Build history of the part. All positions in model axes, mm. Face numbers are marked on the shaded views. A direction names the side the tool comes from. Round coordinates to 2 decimals unless told otherwise and drop trailing zeros. Loops run counter-clockwise (first coordinate to the right, second up) from the corner with the lowest first, then second, coordinate; pieces in that order, holes last. Notation, with made-up numbers: (76.25, 35.5) -> (80.25, 35.5) arc R15 cw to (80.25, 45.5) -> close; hole circle Ø6 at (83.5, 82.25). An arc over 180 degrees is marked (long way). Put each result on its own line as item: value. Start each with the question number.
```python
from build123d import *

# Parameters (mm, degrees)
SKETCH1_W           = 80
SKETCH1_H           = 65.45
BOSS_EXTRUDE1_DEPTH = 31
BOSS_EXTRUDE3_DEPTH = 5
CHAMFER2_SIZE       = 25
CHAMFER2_SIZE2      = 20.977490779
SHELL2_START        = -36
SHELL2_DEPTH        = 72
SHELL2_START_2      = -41
SHELL2_2_OUTLINE_W  = 1
SHELL2_2_OUTLINE_H  = 57.45
SHELL2_2_DEPTH      = 82
SKETCH6_R           = 4.86874318
CUT_EXTRUDE1_DEPTH  = 5
BOSS_EXTRUDE4_DEPTH = 8
BOSS_EXTRUDE5_REACH = 107.939
BOSS_EXTRUDE5_START = 29.5
SKETCH10_W          = 12.25
SKETCH10_H          = 9
CUT_EXTRUDE2_DEPTH  = 6
CHAMFER3_SIZE       = 2
CHAMFER3_SIZE2      = 1.865030172
CHAMFER4_SIZE       = 7.098078142
CHAMFER4_SIZE_2     = 10
CHAMFER5_SIZE       = 10
CHAMFER7_SIZE       = 5
SKETCH11_R          = 0.93
CUT_EXTRUDE3_DEPTH  = 7


# Read off the part's stored shape, not the designer's step: Shell2
with BuildPart() as part:
    # Sketch1 → Boss-Extrude1 (new body)
    with BuildSketch(Plane(origin=(0, 0, 0), x_dir=(1, 0, 0), z_dir=(0, 1, 0))):
        Rectangle(SKETCH1_W, SKETCH1_H)
    extrude(amount=BOSS_EXTRUDE1_DEPTH)

    # Sketch5 → Boss-Extrude3 (add)
    with BuildSketch(Plane.ZY.offset(40)):
        Polygon((-32.725, 31), (-20.625, 31), (8.005, 31), (32.725, 31), (32.725, 26), (2.6203214, 26), (6.0203214, 22.6), (-5.2796786, 22.6), (-1.8796786, 26), (-16.125, 26), (-12.725, 22.6), (-24.025, 22.6), (-20.625, 26), (-32.725, 26), align=None)
    boss_extrude3 = extrude(amount=BOSS_EXTRUDE3_DEPTH)

    # Mirror1: Boss-Extrude3 across plane
    add(boss_extrude3.mirror(Plane(origin=(0, 0, 0), x_dir=(0, 0, 1), z_dir=(1, 0, 0))))

    # Chamfer2
    chamfer2_edges = [part.edges().sort_by_distance(p)[0] for p in [
        (0, 0, 32.725),
    ]]
    chamfer2_side = [part.faces().sort_by_distance(p)[0] for p in [
        (0, 0, 0),
    ]]
    chamfer(chamfer2_edges, length=CHAMFER2_SIZE, length2=CHAMFER2_SIZE2, reference=chamfer2_side[0])

    # Shell2 outline → Shell2 (cut)
    with BuildSketch(Plane.YZ.offset(SHELL2_START)):
        Polygon((22.842721412, 28.725), (4, 6.269119063), (4, -28.725), (31, -28.725), (31, 28.725), align=None)
    extrude(amount=SHELL2_DEPTH, mode=Mode.SUBTRACT)

    # Shell2 2 outline → Shell2 2 (cut)
    with BuildSketch(Plane.YZ.offset(SHELL2_START_2)):
        with Locations((30.5, 0)):
            Rectangle(SHELL2_2_OUTLINE_W, SHELL2_2_OUTLINE_H)
    extrude(amount=SHELL2_2_DEPTH, mode=Mode.SUBTRACT)

    # Sketch6 → Cut-Extrude1 (cut)
    with BuildSketch(Plane(origin=(0, 4, 24.632603001), x_dir=(1, 0, 0), z_dir=(0, 1, 0))):
        with Locations(Location((22, 23.453346141, 0), (0, 0, 270))):
            Circle(SKETCH6_R)
        with Locations(Location((-22, 23.453346141, 0), (0, 0, 270))):
            Circle(SKETCH6_R)
    extrude(amount=-CUT_EXTRUDE1_DEPTH, mode=Mode.SUBTRACT)

    # Sketch7 → Boss-Extrude4 (add)
    with BuildSketch(Plane.XY.offset(-28.725)):
        Polygon((-14.5, 13.5), (14.5, 13.5), (14.5, 31), (13.5, 31), (13.5, 14.706896552), (-13.5, 14.706896552), (-13.5, 31), (-14.5, 31), align=None)
    extrude(amount=BOSS_EXTRUDE4_DEPTH)

    # Sketch8 → Boss-Extrude5 (add, up to next)
    with BuildSketch(Plane.XY.offset(-20.725).offset(BOSS_EXTRUDE5_START), mode=Mode.PRIVATE) as boss_extrude5_sk1:
        Polygon((-13.5, 14.706896552), (-13.5, 31), (-14.5, 31), (-14.5, 14.706896552), (-14.5, 13.5), (-13.5, 13.5), (13.5, 13.5), (14.5, 13.5), (14.5, 14.706896552), (14.5, 31), (13.5, 31), (13.5, 14.706896552), align=None)
    boss_extrude5_tool1 = extrude(boss_extrude5_sk1.sketch, amount=BOSS_EXTRUDE5_REACH, mode=Mode.PRIVATE) - part.part
    add(boss_extrude5_tool1.solids().sort_by_distance((14, 30.661289, 8.775))[0])

    # Sketch10 → Cut-Extrude2 (cut)
    with BuildSketch(Plane.XZ):
        with Locations((-26.125, -23.025)):
            Rectangle(SKETCH10_W, SKETCH10_H)
        with Locations((26.125, -23.025)):
            Rectangle(SKETCH10_W, SKETCH10_H)
    extrude(amount=-CUT_EXTRUDE2_DEPTH, mode=Mode.SUBTRACT)

    # Chamfer3
    chamfer3_edges = [part.edges().sort_by_distance(p)[0] for p in [
        (0, 31, -32.725),
    ]]
    chamfer3_side = [part.faces().sort_by_distance(p)[0] for p in [
        (0, 15.756916996, -32.725),
    ]]
    chamfer(chamfer3_edges, length=CHAMFER3_SIZE, length2=CHAMFER3_SIZE2, reference=chamfer3_side[0])

    # Chamfer4
    # the kernel refuses this chamfer: 10, 7.098078142 mm, written as the material it adds along each edge
    with BuildSketch(Plane(origin=(14.5, 13.5, 17.590778193), x_dir=(0, -0.6849156240265527, -0.728622390518105), z_dir=(-1, 0, 0))) as chamfer4_piece_1_section:
        Polygon((CHAMFER4_SIZE * 0.998412410217, -CHAMFER4_SIZE * 0.0563263630269), (CHAMFER4_SIZE_2 * 0.728622390518, -CHAMFER4_SIZE_2 * 0.684915624027), (0, 0), align=None)
    chamfer4_piece_1 = extrude(amount=29, mode=Mode.PRIVATE)
    chamfer4_piece_1 = split(chamfer4_piece_1, bisect_by=Plane(origin=(0, 11.943437141, 8.775), z_dir=(0, 0, 1)), keep=Keep.TOP, mode=Mode.PRIVATE)
    add(chamfer4_piece_1)

    # Chamfer5
    # the kernel refuses this chamfer: 10 mm, written as the material it adds along each edge
    with BuildSketch(Plane(origin=(-14.5, 13.5, -28.725), x_dir=(0, 0.027495876610586317, 0.9996219169112968), z_dir=(1, 0, 0))) as chamfer5_piece_1_section:
        Polygon((CHAMFER5_SIZE * 0.999621916911, CHAMFER5_SIZE * 0.0274958766106), (-CHAMFER5_SIZE * 0.0274958766106, CHAMFER5_SIZE * 0.999621916911), (0, 0), align=None)
    chamfer5_piece_1 = extrude(amount=29, mode=Mode.PRIVATE)
    chamfer5_piece_1 = split(chamfer5_piece_1, bisect_by=Plane(origin=(0, 10.042815877, -20.725), z_dir=(0, 0, -1)), keep=Keep.TOP, mode=Mode.PRIVATE)
    add(chamfer5_piece_1)

    # Chamfer7
    chamfer7_edges = [part.edges().sort_by_distance(p)[0] for p in [
        (40, 10.48874539, 20.225),
        (-40, 10.48874539, 20.225),
        (-40, 13, -32.725),
        (40, 13, -32.725),
    ]]
    chamfer(chamfer7_edges, length=CHAMFER7_SIZE)

    # Sketch11 → Cut-Extrude3 (cut)
    with BuildSketch(Plane(origin=(0, 30, 0), x_dir=(1, 0, 0), z_dir=(0, 1, 0))):
        with Locations(Location((38.849613738, -26.574613738, 0), (0, 0, 270))):
            Circle(SKETCH11_R)
        with Locations(Location((38.849613738, 26.574613738, 0), (0, 0, 90))):
            Circle(SKETCH11_R)
        with Locations(Location((-38.849613738, 26.574613738, 0), (0, 0, 270))):
            Circle(SKETCH11_R)
        with Locations(Location((-38.849613738, -26.574613738, 0), (0, 0, 90))):
            Circle(SKETCH11_R)
    extrude(amount=-CUT_EXTRUDE3_DEPTH, mode=Mode.SUBTRACT)


solid = part.part
```
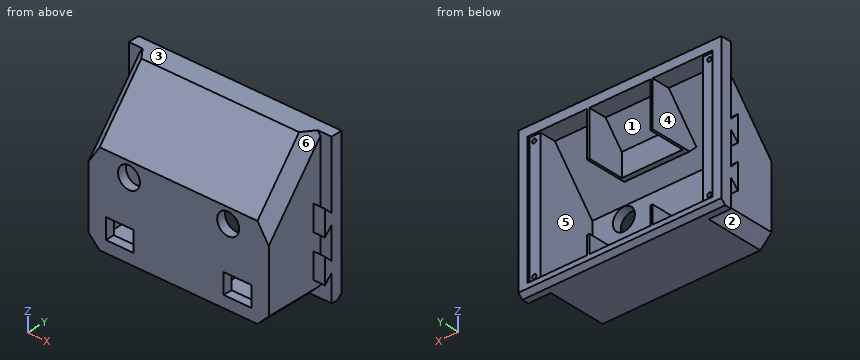
Item 1: Cut at B-B on x = -6.5. Write the cut outline in (y, z) (1 decimal).
Item 2: Pull direction X, two halves, no side cores. Call the marked faces 1, 2, 3 and 4: +X half, -X half, draft (parallel to the pull), parting line (faces both ways), or undercut.
Item 3: Drop flat-ended pins along their axis: pin 1 (2.5 mm diameter, centred on x = -42, z = -18.5, fed in from -Y); pin 2 (12 mm diameter, centred on y = 8.5, z = 22.5, fed in from +X); pin 3 (4 mm diameter, centred on x = -35, z = -11, fed in from +Y). Give the stop position or say it passes through.
Item 4: Cut at A-A on x = -22. State how many separate pieces and enclosed holes the cut face has, then the cut area to 3 significant figures.
Item 5: Wall check: line 1 (X direction, y = 19.5, z = -22); line 2 (X direction, y = 14, z = 11.5); line 3 (X direction, y = 20.5, z = 0). Give the ranges that are in metal, low to high. Write a range as from..to.
Item 6: Cut at D-D on z = 16. Write the cut outline in (x, y).
Item 7: 3-axis set-ups, long thin cutter, end or side, ignore diameter. For the marked faces 5 and 6: which of +Z, -Z, +X, -X, +Y, -Y reach the whole face in a straight line?
Item 8: Cut at C-C on y = 18. Write the cut outline in (x, z) (3 decimals).
Ans:
1. outline: (0, -32.7) -> (29, -32.7) -> (31, -30.9) -> (31, -28.7) -> (14.7, -28.7) -> (14.7, -20.7) -> (11.5, -20.7) -> (4, -28.2) -> (4, 6.3) -> (8.9, 12.2) -> (12.3, 8.8) -> (14.7, 8.8) -> (14.7, 19) -> (22.8, 28.7) -> (31, 28.7) -> (31, 32.7) -> (21, 32.7) -> (0, 7.7) -> close
2. face 1: undercut
2. face 2: -X half
2. face 3: draft
2. face 4: undercut
3. pin 1: stops at y = 22.6
3. pin 2: stops at x = 38.01
3. pin 3: stops at y = 30
4. separate pieces: 3
4. enclosed holes: 0
4. area: 350 mm2
5. line 1: x = -40..-36, -14.5..-13.5, 13.5..14.5, 36..40
5. line 2: x = -40..-36, -14.5..14.5, 36..40
5. line 3: x = -40..-36, 36..40
6. outline: (-45, 26) -> (-40, 26) -> (-40, 13.47) -> (-35, 6.94) -> (35, 6.94) -> (40, 13.47) -> (40, 26) -> (45, 26) -> (45, 31) -> (41, 31) -> (41, 30) -> (36, 30) -> (36, 12.17) -> (14.5, 12.17) -> (14.5, 31) -> (13.5, 31) -> (13.5, 14.71) -> (-13.5, 14.71) -> (-13.5, 31) -> (-14.5, 31) -> (-14.5, 12.17) -> (-36, 12.17) -> (-36, 30) -> (-41, 30) -> (-41, 31) -> (-45, 31) -> close
7. face 5: +Y
7. face 6: +Z, +X, -Y
8. outline: (-40, -27.725) -> (-35, -32.725) -> (35, -32.725) -> (40, -27.725) -> (40, 21.398) -> (35, 29.177) -> (-35, 29.177) -> (-40, 21.398) -> close; hole (-36, -28.725) -> (-14.5, -28.725) -> (-14.5, -20.725) -> (-13.5, -20.725) -> (-13.5, -28.725) -> (13.5, -28.725) -> (13.5, -20.725) -> (14.5, -20.725) -> (14.5, -28.725) -> (36, -28.725) -> (36, 22.954) -> (14.5, 22.954) -> (14.5, 8.775) -> (13.5, 8.775) -> (13.5, 22.954) -> (-13.5, 22.954) -> (-13.5, 8.775) -> (-14.5, 8.775) -> (-14.5, 22.954) -> (-36, 22.954) -> close
